```python
from build123d import *

# Parameters (mm, degrees)
SKETCH1_W           = 180
SKETCH1_H           = 140
BOSS_EXTRUDE1_DEPTH = 12
SKETCH2_W           = 62
SKETCH2_H           = 112
CUT_EXTRUDE1_DEPTH  = 9
SKETCH3_R           = 7.5
BOSS_EXTRUDE2_DEPTH = 10
SKETCH4_W           = 21.5
SKETCH4_H           = 9.1
CUT_EXTRUDE2_DEPTH  = 229.825260843
FILLET4_R           = 2
FILLET5_R           = 2
FILLET6_R           = 2
FILLET7_R           = 5


with BuildPart() as part:
    # Sketch1 → Boss-Extrude1 (new body)
    with BuildSketch(Plane.XY):
        with Locations((90, -70)):
            Rectangle(SKETCH1_W, SKETCH1_H)
    extrude(amount=BOSS_EXTRUDE1_DEPTH)

    # Sketch2 → Cut-Extrude1 (cut)
    with BuildSketch(Plane(origin=(0, 0, 0), x_dir=(-1, 0, 0), z_dir=(0, 0, -1))):
        with Locations((-125, -70)):
            Rectangle(SKETCH2_W, SKETCH2_H)
        with Locations((-55, -70)):
            Rectangle(SKETCH2_W, SKETCH2_H)
    extrude(amount=-CUT_EXTRUDE1_DEPTH, mode=Mode.SUBTRACT)

    # Sketch3 → Boss-Extrude2 (add)
    with BuildSketch(Plane(origin=(0, 0, 0), x_dir=(-1, 0, 0), z_dir=(0, 0, -1))):
        with Locations(Location((-168, -13, 0), (0, 0, 180))):
            Circle(SKETCH3_R)
        with Locations(Location((-12, -13, 0), (0, 0, 180))):
            Circle(SKETCH3_R)
        with Locations(Location((-12, -127, 0), (0, 0, 180))):
            Circle(SKETCH3_R)
        with Locations(Location((-168, -127, 0), (0, 0, 180))):
            Circle(SKETCH3_R)
    extrude(amount=BOSS_EXTRUDE2_DEPTH)

    # Sketch4 → Cut-Extrude2 (cut, through all)
    with BuildSketch(Plane(origin=(0, 0, 9), x_dir=(-1, 0, 0), z_dir=(0, 0, -1))):
        with Locations((-108.35, -20.85)):
            Rectangle(SKETCH4_W, SKETCH4_H)
        with Locations((-38.35, -20.85)):
            Rectangle(SKETCH4_W, SKETCH4_H)
    extrude(amount=-CUT_EXTRUDE2_DEPTH, mode=Mode.SUBTRACT)

    # Fillet4
    fillet4_edges = [part.edges().sort_by_distance(p)[0] for p in [
        (119.1, -16.3, 10.5),
    ]]
    fillet(fillet4_edges, radius=FILLET4_R)

    # Fillet5
    fillet5_edges = [part.edges().sort_by_distance(p)[0] for p in [
        (119.1, -25.4, 10.5),
        (97.6, -16.3, 10.5),
        (97.6, -25.4, 10.5),
    ]]
    fillet(fillet5_edges, radius=FILLET5_R)

    # Fillet6
    fillet6_edges = [part.edges().sort_by_distance(p)[0] for p in [
        (49.1, -25.4, 10.5),
        (49.1, -16.3, 10.5),
        (27.6, -16.3, 10.5),
        (27.6, -25.4, 10.5),
    ]]
    fillet(fillet6_edges, radius=FILLET6_R)

    # Fillet7
    fillet7_edges = [part.edges().sort_by_distance(p)[0] for p in [
        (0, 0, 6),
        (180, 0, 6),
        (180, -140, 6),
        (0, -140, 6),
    ]]
    fillet(fillet7_edges, radius=FILLET7_R)


solid = part.part
```
Part model, mm, in its own coordinate system. A direction names the side the tool comes from. Round coordinates to 2 decimals unless told otherwise and drop trailing zeros. Loops run counter-clockwise (first coordinate to the right, second up) from the corner with the lowest first, then second, coordinate; pieces in that order, holes last.
Item 1: Cut at C-C, the plane z = -6.75. Give the cut face in (x, y), then the cut area to 3 significant figures.
Item 2: 3-axis set-ups, long thin cutter, end or side, ignore diameter. For faces 1 (the face through (55, -126, 4)), 2 (the face through (89, -69, 12)): which of +Z, -Z, +X, -X, +Y, -Y reach the whole face in a straight line?
Item 3: Mould opens along Y. For faces 3 (the face through (12, -13, -10)), 4 (the face through (1, -138, 6)), 5 (the face through (125, -14, 4)) say: +Y half, -Y half, draft (parallel to the pull), parting line (faces both ways), or undercut.
Item 4: Cut at D-D, the plane z = 4. Give the cut face in (x, y).
Item 5: Cut at A-A, the plane x = 168. Give the cut face in (y, z), then the cut area to 3 significant figures.
Item 6: Drop flat-ended pins along their axis: P1, Ø2, axis at x = 81.5, y = -81.5, coming from the -Z side; P2, Ø4, axis at x = 87, z = -2.5, coming from the -Y side. Give the stop position or say it passes through.
Item 7: Cut at B-B, the plane y = -103.5. Give the cut face in (x, z).
Item 8: Drill centre lines: line 1 (X direction, y = -50.5, z = 5); line 2 (Y direction, x = 95.5, z = 0.5); line 3 (Z direction, x = 9.5, y = -40.5). Where is each one in solid material? Low to high.
A:
1. outline: circle Ø15 at (12, -127); circle Ø15 at (12, -13); circle Ø15 at (168, -127); circle Ø15 at (168, -13)
1. area: 707 mm2
2. face 1: -Z
2. face 2: +Z, +X, -X, +Y, -Y
3. face 3: draft
3. face 4: -Y half
3. face 5: undercut
4. outline: (0, -135) arc R5 ccw to (5, -140) - (175, -140) arc R5 ccw to (180, -135) - (180, -5) arc R5 ccw to (175, 0) - (5, 0) arc R5 ccw to (0, -5) - close; hole (24, -126) - (86, -126) - (86, -14) - (24, -14) - close; hole (94, -126) - (156, -126) - (156, -14) - (94, -14) - close
5. outline: (-140, 0) - (-134.5, 0) - (-134.5, -10) - (-119.5, -10) - (-119.5, 0) - (-20.5, 0) - (-20.5, -10) - (-5.5, -10) - (-5.5, 0) - (0, 0) - (0, 12) - (-140, 12) - close
5. area: 1,980 mm2
6. P1: stops at z = 9
6. P2: passes through
7. outline: (0, 0) - (24, 0) - (24, 9) - (86, 9) - (86, 0) - (94, 0) - (94, 9) - (156, 9) - (156, 0) - (180, 0) - (180, 12) - (0, 12) - close
8. line 1: x = 0 to 24, 86 to 94, 156 to 180
8. line 2: y = -140 to -126, -14 to 0
8. line 3: z = 0 to 12
